```python
from build123d import *

# Parameters (mm, degrees)
SKETCH6_R                      = 42.5
SKETCH6_R_2                    = 29
CUT_EXTRUDE3_DEPTH             = 10
SKETCH7_W                      = 10
SKETCH7_H                      = 7.550043706
CUT_EXTRUDE4_DEPTH             = 10
CIRPATTERN2_COUNT              = 3
DELETEFACE1_START              = 15
DELETEFACE1_OUTLINE_R          = 76.2
DELETEFACE1_OUTLINE_R_2        = 55
DELETEFACE1_DEPTH              = 20
F_3_8_CLEARANCE_HOLE1_D        = 9.8044
SKETCH46_R                     = 10
CUT_EXTRUDE5_DEPTH             = 10
CIRPATTERN6_COUNT              = 3
FILLET2_R                      = 3
CIRPATTERN7_COUNT              = 6
F_1_4_0_2500_DOWEL_HOLE1_D     = 6.35
F_1_4_0_2500_DOWEL_HOLE1_DEPTH = 9.906
F_1_4_0_2500_DOWEL_HOLE1_TIP   = 1.907732465


# Read off the part's stored shape, not the designer's step: DeleteFace1
with BuildPart() as part:
    # Sketch3 → Revolve1 (revolve)
    with BuildSketch(Plane(origin=(0, 0, 0), x_dir=(0, 0, -1), z_dir=(1, 0, 0))):
        with BuildLine():
            Line((76.2, 15), (55, 15))
            Line((55, 15), (55, 35))
            Line((55, 35), (22.025, 35))
            Line((22.025, 35), (22.025, 20.36))
            Line((22.025, 20.36), (11.665, 10))
            Line((11.665, 10), (11.665, 0))
            Line((11.665, 0), (16.665, 0))
            ThreePointArc((16.665, 0), (37.471852779, 3.234070807), (53.85, -10))
            Line((53.85, -10), (76.2, -10))
            Line((76.2, -10), (76.2, 15))
        make_face()
    revolve(axis=Axis((0, 0, 0), (0, 1, 0)))

    # Sketch6 → Cut-Extrude3 (cut)
    with BuildSketch(Plane(origin=(0, 35, 0), x_dir=(1, 0, 0), z_dir=(0, 1, 0))):
        with Locations(Location((0, 0, 0), (0, 0, 270))):
            Circle(SKETCH6_R)
        with Locations(Location((0, 0, 0), (0, 0, 270))):
            Circle(SKETCH6_R_2, mode=Mode.SUBTRACT)
    extrude(amount=-CUT_EXTRUDE3_DEPTH, mode=Mode.SUBTRACT)

    # Sketch7 → Cut-Extrude4 (cut)
    with BuildSketch(Plane(origin=(0, 35, 0), x_dir=(1, 0, 0), z_dir=(0, 1, 0))):
        with Locations((0, 25.224978147)):
            Rectangle(SKETCH7_W, SKETCH7_H)
    cut_extrude4 = extrude(amount=-CUT_EXTRUDE4_DEPTH, mode=Mode.SUBTRACT)

    # CirPattern2: Cut-Extrude4 ×3 about axis
    cirpattern2_axis = Axis((0, 0, 0), (0, 1, 0))
    for i in range(1, CIRPATTERN2_COUNT):
        add(cut_extrude4.rotate(cirpattern2_axis, i * 360 / CIRPATTERN2_COUNT), mode=Mode.SUBTRACT)

    # DeleteFace1 outline → DeleteFace1 (add)
    with BuildSketch(Plane(origin=(0, 0, 0), x_dir=(1, 0, 0), z_dir=(0, 1, 0)).offset(DELETEFACE1_START)):
        Circle(DELETEFACE1_OUTLINE_R)
        Circle(DELETEFACE1_OUTLINE_R_2, mode=Mode.SUBTRACT)
    extrude(amount=DELETEFACE1_DEPTH)

    # 3/8 Clearance Hole1 (through all)
    with Locations(Plane(origin=(0, -10, 0), x_dir=(-1, 0, 0), z_dir=(0, -1, 0))):
        with Locations((46.153593538, 46.060907757), (65.203960939, -0.061814491), (46.060915247, -46.146148146), (-0.061807016, -65.196515566), (-46.146140681, -46.053469867), (-65.196508083, 0.069252405), (-46.053462365, 46.15358606), (0.069259897, 65.203953456)):
            Hole(F_3_8_CLEARANCE_HOLE1_D / 2)

    # Sketch46 → Cut-Extrude5 (cut)
    with BuildSketch(Plane(origin=(0, 35, 0), x_dir=(1, 0, 0), z_dir=(0, 1, 0))):
        with Locations((41.099239846, 12.958540547)):
            Circle(SKETCH46_R)
    cut_extrude5 = extrude(amount=-CUT_EXTRUDE5_DEPTH, mode=Mode.SUBTRACT)

    # CirPattern6: Cut-Extrude5 ×3 about axis
    cirpattern6_axis = Axis((0, 0, 0), (0, 1, 0))
    for i in range(1, CIRPATTERN6_COUNT):
        add(cut_extrude5.rotate(cirpattern6_axis, i * 360 / CIRPATTERN6_COUNT), mode=Mode.SUBTRACT)

    # Fillet2
    fillet2_edges = [part.edges().sort_by_distance(p)[0] for p in [
        (36.469652208, 30, -21.822338734),
        (42.390969445, 30, -3.042319763),
        (-37.133525818, 30, -20.672475912),
        (-23.830210924, 30, -35.190496549),
        (0.66387361, 30, 42.494814646),
        (-18.560758521, 30, 38.232816312),
        (5, 30, -28.565713714),
        (-5, 30, -28.565713714),
        (27.238633754, 30, 9.952729838),
        (22.238633754, 30, 18.612983876),
        (-22.238633754, 30, 18.612983876),
        (-27.238633754, 30, 9.952729838),
    ]]
    fillet(fillet2_edges, radius=FILLET2_R)

    # Sketch51 → 1/4-28 Tapped Hole1 (revolve, cut)
    with BuildSketch(Plane(origin=(25.5125, 35, 0), x_dir=(0, 0, 1), z_dir=(1, 0, 0))):
        Polygon((0, 0), (0, 17.045388061), (2.7051, 15.42), (2.7051, 0), align=None)
    f_1_4_28_tapped_hole1 = revolve(axis=Axis((25.5125, 41.35, 0), (0, -1, 0)), mode=Mode.SUBTRACT)

    # CirPattern7: 1/4-28 Tapped Hole1 ×6 about axis, 2 skipped
    cirpattern7_axis = Axis((0, 0, 0), (0, -1, 0))
    add([f_1_4_28_tapped_hole1.rotate(cirpattern7_axis, i * 360 / CIRPATTERN7_COUNT) for i in range(1, CIRPATTERN7_COUNT) if i not in (2, 5)], mode=Mode.SUBTRACT)

    # 1/4 (0.2500) Dowel Hole1
    with Locations(Plane(origin=(0, -10, 0), x_dir=(-1, 0, 0), z_dir=(0, -1, 0))):
        with Locations((-25.007850676, -60.207814752), (25.01513322, 60.21585851)):
            Hole(F_1_4_0_2500_DOWEL_HOLE1_D / 2, depth=F_1_4_0_2500_DOWEL_HOLE1_DEPTH)
            with Locations((0, 0, -(F_1_4_0_2500_DOWEL_HOLE1_DEPTH + F_1_4_0_2500_DOWEL_HOLE1_TIP / 2))):  # 118° drill point
                Cone(0, F_1_4_0_2500_DOWEL_HOLE1_D / 2, F_1_4_0_2500_DOWEL_HOLE1_TIP, mode=Mode.SUBTRACT)


solid = part.part
```
Verification items for the finished model (mm, model axes). A direction names the side the tool comes from. Round coordinates to 2 decimals unless told otherwise and drop trailing zeros. Write each question's results on one line, items separated by ' | '.
Q1. Sectioned sample at A-A, the plane y = 29.5. Give the number of separate pieces and of enclosed holes in the cut face, and give its area (3 significant figures).
Derived:
separate pieces: 4 | enclosed holes: 13 | area: 12,200 mm²
Q2. Thickness scan on probe 1 along X at (y, z) = (28.5, -4); probe 2 along X at (y, z) = (-8, 3.5); probe 3 along Z at (x, y) = (9, 28). Record the ranges inside material, lowest first.
Derived:
probe 1: x = -76.09 to -67.95, -62.46 to -42.31, -28.72 to -21.66, 21.66 to 28.72, 45.54 to 62.27, 68.13 to 76.09 | probe 2: x = -76.12 to -68.7, -61.71 to -52.59, 52.59 to 61.84, 68.56 to 76.12 | probe 3: z = -75.67 to -41.54, -27.57 to -20.1, 20.1 to 27.57, 41.54 to 75.67
Q3. Draft check along X on faces 1 (the face through (-17.3, -10, -51.2)), 2 (the face through (0, 30, 29)). Enter one of: released by +X, released by -X, zero draft, split by the parting line, or undercut.
Derived:
face 1: zero draft | face 2: undercut
Q4. Go/stop test with flat-tipped pins: pin 1 Ø5 at (x, y) = (-16, -4) entering from -Z; pin 2 Ø8 at (x, z) = (-46.06, 46.15) entering from -Y; pin 3 Ø2 at (x, z) = (-23, 12) entering from -Y; pin 4 Ø6 at (x, z) = (-25.51, 0) entering from -Y. Record where each tip stops, or that it passes through.
Derived:
pin 1: stops at z = -74.99 | pin 2: passes through | pin 3: stops at y = 3.48 | pin 4: stops at y = 2.8
Q5. Access from +Z, -Z, +X, -X, +Y, -Y to the whole of each face (thin tool, end or side, straight path). Record for faces 3 (the face through (-1.001, 12.815, 69.982)), 4 (the face through (-38.998, 30.07, -36.026)).
Derived:
face 3: +Y, -Y | face 4: +Y
